```python
from build123d import *

# Parameters (mm, degrees)
EXTRUDE_THIN1_START = 160.5026
SKETCH3_R           = 55.2
SKETCH3_R_2         = 55
EXTRUDE_THIN1_DEPTH = 160.5026


with BuildPart() as part:
    # Sketch2 → Revolve2 (revolve)
    with BuildSketch(Plane.XY, mode=Mode.PRIVATE) as revolve2_sk:
        with BuildLine():
            Line((0, -51), (0, -65))
            Line((0, -65), (3.5, -65))
            ThreePointArc((3.5, -65), (5, -63.5), (6.5, -65))
            Line((6.5, -65), (12, -65))
            Line((12, -65), (12, -62.5))
            Line((12, -62.5), (10.5, -62.5))
            Line((10.5, -62.5), (10.5, -55))
            Line((10.5, -55), (26, -55))
            Line((26, -55), (26, -56.3))
            Line((26, -56.3), (30, -56.3))
            Line((30, -56.3), (30, -51))
            Line((30, -51), (0, -51))
        make_face()
    revolve2 = revolve(revolve2_sk.sketch.rotate(Axis((400.5834, 0, 0), (-1, 0, 0)), 270), axis=Axis((400.5834, 0, 0), (-1, 0, 0)))

    # Sketch3 → Extrude-Thin1 (add)
    with BuildSketch(Plane(origin=(30, 0, 0), x_dir=(0, 0, -1), z_dir=(1, 0, 0)).offset(EXTRUDE_THIN1_START)):
        Circle(SKETCH3_R)
        Circle(SKETCH3_R_2, mode=Mode.SUBTRACT)
    extrude_thin1 = extrude(amount=-EXTRUDE_THIN1_DEPTH)

    # Mirror1: Revolve2, Extrude-Thin1 across plane
    add(revolve2.mirror(Plane(origin=(190.5026, 0, 0), x_dir=(0, 0, 1), z_dir=(1, 0, 0))))
    add(extrude_thin1.mirror(Plane(origin=(190.5026, 0, 0), x_dir=(0, 0, 1), z_dir=(1, 0, 0))))


solid = part.part
```
Source: CAD feature listing. Evaluate the final solid. Frame: model axes, mm. A direction names the side the tool comes from. Round coordinates to 2 decimals unless told otherwise and drop trailing zeros. Loops run counter-clockwise (first coordinate to the right, second up) from the corner with the lowest first, then second, coordinate; pieces in that order, holes last.
(1) Pull-direction query (X, two-part tool) for faces 3 (the flat face through (370.505, 55.3, 0.3)), 4 (the cylindrical face through (371.72, -19.52, -62)), 5 (the flat face through (0, 33.4, -38.8)); classes: +X half, -X half, draft (parallel to the pull), parting line (faces both ways), or undercut.
From the geometry:
face 3: undercut
face 4: draft
face 5: -X half
(2) Contact query for flat-ended pins moving along their axis: pin 1 Ø4 at (x, z) = (235.5, -16.5) entering from -Y; pin 2 Ø5 at (x, y) = (89.5, 9) entering from -Z; pin 3 Ø5 at (x, z) = (290.5, 8) entering from -Y; pin 4 Ø10 at (y, z) = (-43.5, 11) entering from +X. Output: stop coordinate, or through.
From the geometry:
pin 1: stops at y = -53.26
pin 2: stops at z = -54.82
pin 3: stops at y = -54.93
pin 4: passes through
(3) Section query A-A (x = 150.5). Output: boundary loops of the cut face in (y, z), and give its area (3 significant figures).
From the geometry:
outline: circle Ø110.4 at (0, 0); hole circle Ø110 at (0, 0)
area: 69.2 mm2
(4) Access query for faces 1 (the cylindrical face through (366.215, 49.787, 11.056)), 2 (the cylindrical face through (369.77, -2.75, 62.44)). Directions: +Z, -Z, +X, -X, +Y, -Y. A direction counts if a zero-diameter tool reaches every point of the face in a straight line with its end or side. Return the directions, or none.
From the geometry:
face 1: +X, -X
face 2: none
(5) Material intervals for probe 1 along Y at (x, z) = (11.15, 0); probe 2 along Y at (x, z) = (247.5, 0); probe 3 along X at (y, z) = (-22.5, 48), sorted ascending.
From the geometry:
probe 1: y = -65 to -62.5, -55 to -51, 51 to 55, 62.5 to 65
probe 2: y = -55.2 to -55, 55 to 55.2
probe 3: x = 0 to 30, 351.01 to 381.01
